Check sheet for the drawn part. Datum: minimum x, y, z corner. Units: mm. Give positions to 0.01 mm unless a question says otherwise; leave off trailing zeros. Write each loop counter-clockwise with the first axis right and the second up, starting at its lowest first coordinate (ties: lowest second). Pieces come first, ordered by that corner, then holes. Notation, with made-up numbers: (29.25, 39) -> (74.25, 39) arc R20 cw to (74.25, 49) -> close; hole circle Ø8 at (10, -15.75). An arc over 180 degrees is marked (long way). Use CSV: the item, a comma, the result in double quotes. Start each with the question number.
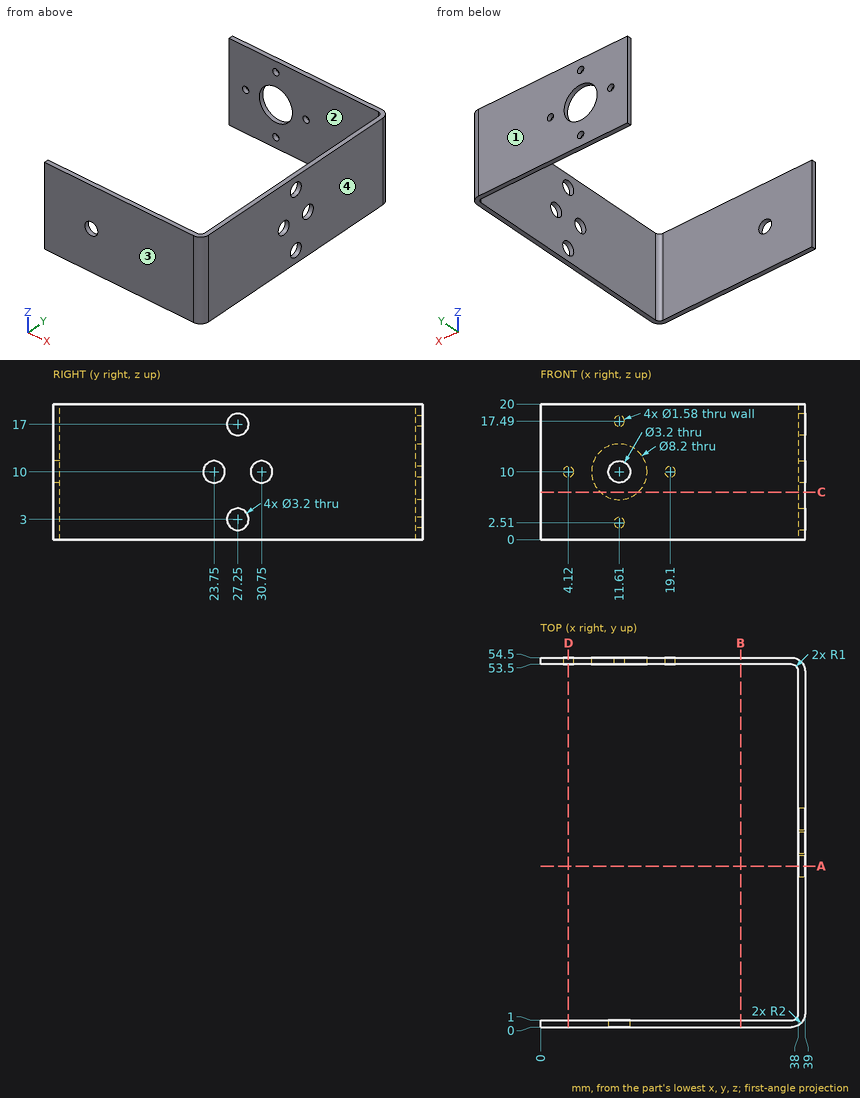
(1) Section check B-B on x = 29.5. Record the cut outline in (y, z).
(2) Thickness scan on line 1 (Z direction, x = 11.61, y = 54.05); line 2 (Y direction, x = 37, z = 11.25); line 3 (Y direction, x = 38.4, z = 10). Record the ranges inside material, lowest first. Write a range as from..to.
(3) Section check C-C on z = 7. Record the cut outline in (x, y).
(4) Go/stop test with flat-tipped pins: pin 1 (4 mm diameter, centred on y = 43, z = 14.5, fed in from -X); pin 2 (5 mm diameter, centred on x = 11.61, z = 10, fed in from +Y). Record where each tip stops, or that it passes through.
(5) Section check D-D on x = 4.12. Record the cut outline in (y, z).
(6) Draft check along Y on the marked faces 1, 2, 3 and 4. Enter one of: released by +Y, released by -Y, zero draft, split by the parting line, or undercut.
(7) Section check A-A on y = 23.75. Record the cut outline in (x, z), then the cut area to 3 significant figures.
Data:
1,outline,"(0, 0) -> (1, 0) -> (1, 20) -> (0, 20) -> close; (53.5, 0) -> (54.5, 0) -> (54.5, 20) -> (53.5, 20) -> close"
2,line 1,"z = 0..1.72, 3.3..5.9, 14.1..16.7, 18.28..20"
2,line 2,"y = 0..1, 53.5..54.5"
2,line 3,"y = 0.57..22.15, 25.35..29.15, 32.35..53.93"
3,outline,"(0, 0) -> (37, 0) arc R2 ccw to (39, 2) -> (39, 52.5) arc R2 ccw to (37, 54.5) -> (14.4, 54.5) -> (14.4, 53.5) -> (37, 53.5) arc R1 cw to (38, 52.5) -> (38, 2) arc R1 cw to (37, 1) -> (0, 1) -> close; (0, 53.5) -> (8.82, 53.5) -> (8.82, 54.5) -> (0, 54.5) -> close"
4,pin 1,"stops at x = 38"
4,pin 2,"stops at y = 1"
5,outline,"(0, 0) -> (1, 0) -> (1, 20) -> (0, 20) -> close; (53.5, 0) -> (54.5, 0) -> (54.5, 9.21) -> (53.5, 9.21) -> close; (53.5, 10.79) -> (54.5, 10.79) -> (54.5, 20) -> (53.5, 20) -> close"
6,face 1,"released by +Y"
6,face 2,"undercut"
6,face 3,"released by -Y"
6,face 4,"zero draft"
7,outline,"(38, 0) -> (39, 0) -> (39, 8.4) -> (38, 8.4) -> close; (38, 11.6) -> (39, 11.6) -> (39, 20) -> (38, 20) -> close"
7,area,"16.8 mm2"
